The listing builds one solid part. Answer for the finished solid, in the listing's coordinates (mm). A direction names the side the tool comes from. Coordinates: 2 decimals unless noted, no trailing zeros. Order: outer loops, then holes, each group sorted by start corner. A loop starts at its lowest first (then second) coordinate and runs counter-clockwise, first axis right, second up. Notation, with made-up numbers: (28.25, 87.25) -> (72.25, 87.25) arc R8 cw to (72.25, 99.25) -> close; hole circle Ø3 at (-39, -22). An arc over 180 degrees is marked (long way). Answer in a Markdown table with one row per item.
```python
from build123d import *

# Parameters (mm, degrees)
SKETCH2_W           = 34.4
SKETCH2_H           = 88.6
BOSS_EXTRUDE1_DEPTH = 2
SKETCH5_R           = 2
CUT_EXTRUDE1_DEPTH  = 2
SKETCH8_W           = 28.4
SKETCH8_H           = 8.173290792
BOSS_EXTRUDE2_DEPTH = 150
SKETCH11_W          = 34.4
SKETCH11_H          = 5
BOSS_EXTRUDE4_DEPTH = 10
SKETCH12_R          = 1.1
CUT_EXTRUDE2_DEPTH  = 50
FILLET1_R           = 40


with BuildPart() as part:
    # Sketch2 → Boss-Extrude1 (new body)
    with BuildSketch(Plane.XY):
        with Locations((142.4072434, -76.6)):
            Rectangle(SKETCH2_W, SKETCH2_H)
    extrude(amount=BOSS_EXTRUDE1_DEPTH)

    # Sketch5 → Cut-Extrude1 (cut)
    with BuildSketch(Plane.XY.offset(2)):
        with Locations((151.0072434, -114.9)):
            Circle(SKETCH5_R)
        with Locations((133.8072434, -114.9)):
            Circle(SKETCH5_R)
        with Locations((133.8072434, -38.3)):
            Circle(SKETCH5_R)
        with Locations((151.0072434, -38.3)):
            Circle(SKETCH5_R)
    extrude(amount=-CUT_EXTRUDE1_DEPTH, mode=Mode.SUBTRACT)

    # Sketch8 → Boss-Extrude2 (add)
    with BuildSketch(Plane.XY.offset(2)):
        Polygon((125.2072434, -57.477141606), (125.2072434, -108.9), (159.6072434, -108.9), (159.6072434, -57.477141606), (156.6072434, -57.477141606), (156.6072434, -65.650432398), (156.6072434, -105.9), (128.2072434, -105.9), (128.2072434, -65.650432398), (128.2072434, -57.477141606), align=None)
        with Locations((142.4072434, -61.563787002)):
            Rectangle(SKETCH8_W, SKETCH8_H)
    extrude(amount=BOSS_EXTRUDE2_DEPTH)

    # Sketch11 → Boss-Extrude4 (add)
    with BuildSketch(Plane.XY.offset(152)):
        with Locations((142.4072434, -111.4)):
            Rectangle(SKETCH11_W, SKETCH11_H)
    extrude(amount=-BOSS_EXTRUDE4_DEPTH)

    # Sketch12 → Cut-Extrude2 (cut)
    with BuildSketch(Plane.XY.offset(152)):
        with Locations((138.33970051, -61.773162564)):
            Circle(SKETCH12_R)
        with Locations((147.28970051, -61.773162564)):
            Circle(SKETCH12_R)
        with Locations((138.33970051, -109.773162564)):
            Circle(SKETCH12_R)
        with Locations((147.28970051, -109.773162564)):
            Circle(SKETCH12_R)
    extrude(amount=-CUT_EXTRUDE2_DEPTH, mode=Mode.SUBTRACT)

    # Fillet1
    # the kernel refuses this fillet: 40 mm, written as the material it adds along each edge
    with BuildSketch(Plane(origin=(125.2072434, -108.9, 142), x_dir=(0, -1, 0), z_dir=(1, 0, 0))) as fillet1_piece_1_section:
        with BuildLine():
            CenterArc((40, 19.364916731), FILLET1_R, 180, 28.955024372)
            Line((0, 19.364916731), (-0.8, 19.364916731))
            Line((-0.8, 19.364916731), (-0.8, 0))
            Line((-0.8, 0), (0, -0.8))
            ThreePointArc((0, -0.8), (2.5, -0.8), (4.3, -0.387298335))
            Line((4.3, -0.387298335), (5, 0))
        make_face()
    fillet1_piece_1 = extrude(amount=60.875729403, mode=Mode.PRIVATE)
    fillet1_piece_1 = split(fillet1_piece_1, bisect_by=Plane(origin=(159.6072434, -109.845330822, 136.09364372), z_dir=(-1, 0, 0)), keep=Keep.TOP, mode=Mode.PRIVATE)
    fillet1_piece_1 = fillet1_piece_1 - Plane(origin=(147.28970051, -109.773162564, 136.09364372), x_dir=(1, 0, 0), z_dir=(0, 0, 1)) * Cylinder(1.1, 200, mode=Mode.PRIVATE)
    fillet1_piece_1 = fillet1_piece_1 - Plane(origin=(138.33970051, -109.773162564, 136.09364372), x_dir=(1, 0, 0), z_dir=(0, 0, 1)) * Cylinder(1.1, 200, mode=Mode.PRIVATE)
    add(fillet1_piece_1)


solid = part.part
```
(1) A cutting plane is placed at D-D, the plane z = 108. Determine the outline of the cut face in (x, y), then the cut area to 3 significant figures.
Check values:
| item | result |
|---|---|
| outline | (125.21, -108.9) -> (137.67, -108.9) arc R1.1 cw to (139.01, -108.9) -> (146.62, -108.9) arc R1.1 cw to (147.96, -108.9) -> (159.61, -108.9) -> (159.61, -57.48) -> (125.21, -57.48) -> close; hole (128.21, -105.9) -> (156.61, -105.9) -> (156.61, -65.65) -> (128.21, -65.65) -> close; hole circle Ø2.2 at (138.34, -61.77); hole circle Ø2.2 at (147.29, -61.77) |
| area | 618 mm² |
(2) A cutting plane is placed at A-A, the plane y = -38.3. Determine the outline of the cut face in (x, z).
Check values:
| item | result |
|---|---|
| outline | (125.21, 0) -> (131.81, 0) -> (131.81, 2) -> (125.21, 2) -> close; (135.81, 0) -> (149.01, 0) -> (149.01, 2) -> (135.81, 2) -> close; (153.01, 0) -> (159.61, 0) -> (159.61, 2) -> (153.01, 2) -> close |
(3) Find the intervals of material crossed by line 1 along Y through (x, z) = (141, 73); line 2 along X through (y, z) = (-97.5, 44.5); line 3 along Y through (x, z) = (147, 137), in increasing order. Write a range as from..to.
Check values:
| item | result |
|---|---|
| line 1 | -108.9..-105.9, -65.65..-57.48 |
| line 2 | 125.21..128.21, 156.61..159.61 |
| line 3 | -111.57..-110.83, -108.71..-105.9, -65.65..-62.83, -60.71..-57.48 |
(4) A cutting plane is placed at C-C, the plane y = -97.5. Determine the outline of the cut face in (x, z), then the cut area to 3 significant figures.
Check values:
| item | result |
|---|---|
| outline | (125.21, 0) -> (159.61, 0) -> (159.61, 152) -> (156.61, 152) -> (156.61, 2) -> (128.21, 2) -> (128.21, 152) -> (125.21, 152) -> close |
| area | 969 mm² |
(5) Which of the six approach directions +Z, -Z, +X, -X, +Y, -Y give full straight-line access (tool end or side, diameter ignored) to faces 1 (the flat face through (143, -57.477, 76)), 2 (the flat face through (142, -85, 2)), 3 (the flat face through (142, -113.9, 147)), 4 (the cylindrical face through (142.166, -110.135, 132.498))?
Check values:
| item | result |
|---|---|
| face 1 | +Z, +X, -X, +Y |
| face 2 | +Z |
| face 3 | +Z, +X, -X, -Y |
| face 4 | +X, -X, -Y |
(6) For a pull along Z with two mould halves and no side action, classify faces 5 (the cylindrical face through (135.655, -39.066, 1.014)), 6 (the flat face through (157, -85, 152)), 7 (the flat face through (142, -115, 2)) as released by +Z, released by -Z, zero draft, split by the parting line, or undercut.
Check values:
| item | result |
|---|---|
| face 5 | zero draft |
| face 6 | released by +Z |
| face 7 | undercut |
(7) A cutting plane is placed at B-B, the plane z = 33.5. Determine the outline of the cut face in (x, y).
Check values:
| item | result |
|---|---|
| outline | (125.21, -108.9) -> (159.61, -108.9) -> (159.61, -57.48) -> (125.21, -57.48) -> close; hole (128.21, -105.9) -> (156.61, -105.9) -> (156.61, -65.65) -> (128.21, -65.65) -> close |
(8) Flat-ended cylindrical pins translate along their axes: pin 1 (4 mm diameter, centred on x = 139.5, y = -89.5, fed in from +Z); pin 2 (6.5 mm diameter, centred on x = 133.81, y = -38.3, fed in from -Z); pin 3 (0.7 mm diameter, centred on x = 138, y = -62, fed in from +Z); pin 4 (5 mm diameter, centred on x = 148, z = 108.5, fed in from -Y). Find the tip coordinate at first contact, or state that the pin passes through.
Check values:
| item | result |
|---|---|
| pin 1 | z = 2 |
| pin 2 | z = 0 |
| pin 3 | z = 102 |
| pin 4 | y = -108.9 |
